Can you work these out from the model? Positions are in its coordinate system, mm. Face numbers are marked on the shaded views. A direction names the side the tool comes from. Coordinates: 2 decimals unless noted, no trailing zeros. Order: outer loops, then holes, each group sorted by start corner. A loop starts at its lowest first (then second) coordinate and runs counter-clockwise, first axis right, second up. Notation, with made-up numbers: (51, -36) -> (83, -36) arc R21 ccw to (83, -3) -> close; hole circle Ø5 at (0, -33). An arc over 180 degrees is marked (long way). Return JSON: item names as keys, results as strings. Group by question number.
1) For pin 1 (19 mm diameter, centred on x = -128.65, z = -36, fed in from -Y); pin 2 (9.5 mm diameter, centred on x = -128.65, z = 36, fed in from +Y); pin 3 (11.5 mm diameter, centred on x = -128.65, z = 36, fed in from +Y); pin 4 (8 mm diameter, centred on x = -128.65, z = -36, fed in from +Y), each with a flat end and sliding along its axis, tell me the tip position at first contact or that it passes through.
2) If we section it at A-A, the plane z = 0: Please give me the cut outline in (x, y), then the cut area to 3 significant figures.
3) If we section it at B-B, the plane y = 35.5: Please give me the cut outline in (x, z).
4) Thinking about a two-plate mould opening in X: for the marked faces 6, 7 and 8, which applies, +X half, -X half, draft (parallel to the pull), parting line (faces both ways), or undercut?
5) If I drill on probe 1 along X at (y, z) = (32.75, -36); probe 2 along X at (y, z) = (10, -36); probe 3 along Z at (x, y) = (-132, 22.5), over which ranges is the centre line in solid material (lowest first)? Write a range as from..to.
6) For the marked faces 1, 2, 3, 4 and 5, which set-ups out of +Z, -Z, +X, -X, +Y, -Y let a thin tool reach every point of the face, with its end or its side?
from build123d import *

# Parameters (mm, degrees)
ESTRUSIONE1_DEPTH                   = 40
SCHIZZO5_R                          = 40.25
ESTRUSIONE4_DEPTH                   = 12.5
SFORMO2_ANGLE                       = 25
RACCORDO1_R                         = 3
RACCORDO2_R                         = 5
RIPETIZIONE_A_L1_COUNT              = 2
RIPETIZIONE_A_L1_PITCH              = 141
SFORMO2_OF_RIPETIZIONE_A_L1_2_ANGLE = 25
RACCORDO1_OF_RIPETIZIONE_A_L1_R     = 3
RACCORDO2_OF_RIPETIZIONE_A_L1_R     = 5
M12_TAPPED_HOLE1_D                  = 10.2
M12_TAPPED_HOLE1_DEPTH              = 32.75
M12_TAPPED_HOLE1_CBORE_D            = 12
M12_TAPPED_HOLE1_CBORE_DEPTH        = 24
M12_TAPPED_HOLE1_TIP                = 3.064389157


with BuildPart() as part:
    # Schizzo2 → Estrusione1 (new body)
    with BuildSketch(Plane(origin=(0, 0, 0), x_dir=(1, 0, 0), z_dir=(0, 1, 0))):
        Polygon((-162.652486086, 21.5), (-162.652486086, -21.5), (-148.652486086, -26.5), (-148.652486086, -66), (-148.652486086, -70), (-144.652486086, -70), (127.347513914, -70), (131.347513914, -70), (131.347513914, -66), (131.347513914, -29.5), (115.347513914, -24.5), (115.347513914, 24.5), (131.347513914, 29.5), (131.347513914, 66), (131.347513914, 70), (127.347513914, 70), (-144.652486086, 70), (-148.652486086, 70), (-148.652486086, 66), (-148.652486086, 26.5), align=None)
    extrude(amount=ESTRUSIONE1_DEPTH)

    # Schizzo5 → Estrusione4 (cut)
    with BuildSketch(Plane.XZ):
        with Locations(Location((-80.652486086, 0, 0), (0, 0, 270))):
            Circle(SCHIZZO5_R)
    estrusione4 = extrude(amount=-ESTRUSIONE4_DEPTH, mode=Mode.SUBTRACT)

    # Sformo2
    sformo2_faces = [part.faces().sort_by_distance(p)[0] for p in [
        (-80.652486086, 6.25, 40.25),
    ]]
    draft(sformo2_faces, Plane(origin=(131.347513914, 0, 29.5), x_dir=(0, 0, -1), z_dir=(0, -1, 0)), SFORMO2_ANGLE)

    # Raccordo1
    raccordo1_edges = [part.edges().sort_by_distance(p)[0] for p in [
        (-80.652486086, 0, 40.25),
    ]]
    fillet(raccordo1_edges, radius=RACCORDO1_R)

    # Raccordo2
    raccordo2_edges = [part.edges().sort_by_distance(p)[0] for p in [
        (-80.652486086, 12.5, 34.421154273),
    ]]
    fillet(raccordo2_edges, radius=RACCORDO2_R)

    # Ripetizione a L1: Estrusione4 ×2
    with Locations(*[(i * RIPETIZIONE_A_L1_PITCH, 0, 0) for i in range(1, RIPETIZIONE_A_L1_COUNT)]):
        add(estrusione4, mode=Mode.SUBTRACT)

    # Sformo2 of Ripetizione a L1 2
    sformo2_of_ripetizione_a_l1_2_faces = [part.faces().sort_by_distance(p)[0] for p in [
        (60.347513914, 6.25, 40.25),
    ]]
    draft(sformo2_of_ripetizione_a_l1_2_faces, Plane(origin=(272.347513914, 0, 29.5), x_dir=(0, 0, -1), z_dir=(0, -1, 0)), SFORMO2_OF_RIPETIZIONE_A_L1_2_ANGLE)

    # Raccordo1 of Ripetizione a L1
    raccordo1_of_ripetizione_a_l1_edges = [part.edges().sort_by_distance(p)[0] for p in [
        (60.347513914, 0, 40.25),
    ]]
    fillet(raccordo1_of_ripetizione_a_l1_edges, radius=RACCORDO1_OF_RIPETIZIONE_A_L1_R)

    # Raccordo2 of Ripetizione a L1
    raccordo2_of_ripetizione_a_l1_edges = [part.edges().sort_by_distance(p)[0] for p in [
        (60.347513914, 12.5, 34.421154273),
    ]]
    fillet(raccordo2_of_ripetizione_a_l1_edges, radius=RACCORDO2_OF_RIPETIZIONE_A_L1_R)

    # M12 Tapped Hole1
    with Locations(Plane(origin=(-128.652486086, 40, -36), x_dir=(0, 0, 1), z_dir=(0, 1, 0))):
        with Locations((0, 0), (0, 230), (72, 230), (72, 0)):
            CounterBoreHole(M12_TAPPED_HOLE1_D / 2, M12_TAPPED_HOLE1_CBORE_D / 2, M12_TAPPED_HOLE1_CBORE_DEPTH, depth=M12_TAPPED_HOLE1_DEPTH)
            with Locations((0, 0, -(M12_TAPPED_HOLE1_DEPTH + M12_TAPPED_HOLE1_TIP / 2))):  # 118° drill point
                Cone(0, M12_TAPPED_HOLE1_D / 2, M12_TAPPED_HOLE1_TIP, mode=Mode.SUBTRACT)


solid = part.part
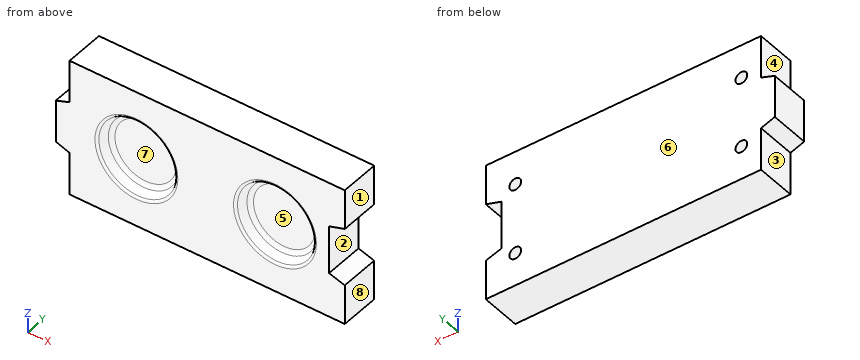
Result sheet:
{
 "1": {"pin 1": "stops at y = 0", "pin 2": "stops at y = 7.04", "pin 3": "stops at y = 16", "pin 4": "stops at y = 6.59"},
 "2": {"outline": "(-162.65, 0) -> (-122.81, 0) arc R3 ccw to (-120.09, 1.73) -> (-116.42, 9.61) arc R5 cw to (-111.89, 12.5) -> (-49.42, 12.5) arc R5 cw to (-44.89, 9.61) -> (-41.21, 1.73) arc R3 ccw to (-38.49, 0) -> (18.19, 0) arc R3 ccw to (20.91, 1.73) -> (24.58, 9.61) arc R5 cw to (29.11, 12.5) -> (91.58, 12.5) arc R5 cw to (96.11, 9.61) -> (99.79, 1.73) arc R3 ccw to (102.51, 0) -> (115.35, 0) -> (115.35, 40) -> (-162.65, 40) -> close", "area": "9,260 mm2"},
 "3": {"outline": "(-162.65, -21.5) -> (-148.65, -26.5) -> (-148.65, -70) -> (131.35, -70) -> (131.35, -29.5) -> (115.35, -24.5) -> (115.35, 24.5) -> (131.35, 29.5) -> (131.35, 70) -> (-148.65, 70) -> (-148.65, 26.5) -> (-162.65, 21.5) -> close; hole circle Ø12 at (-128.65, -36); hole circle Ø12 at (-128.65, 36); hole circle Ø12 at (101.35, -36); hole circle Ø12 at (101.35, 36)"},
 "4": {"face 6": "draft", "face 7": "undercut", "face 8": "+X half"},
 "5": {"probe 1": "x = -148.65..-134.65, -122.65..95.35, 107.35..131.35", "probe 2": "x = -148.65..-133.75, -123.55..96.25, 106.45..131.35", "probe 3": "z = -70..-40.98, -31.02..31.02, 40.98..70"},
 "6": {"face 1": "+Z, -Z, +X, +Y, -Y", "face 2": "+X, +Y, -Y", "face 3": "-Z, -X, +Y, -Y", "face 4": "+Z, -X, +Y, -Y", "face 5": "-Y"}
}
